```python
from build123d import *

# Parameters (mm, degrees)
BASE_W                  = 80
BASE_H                  = 101.6
BOSS_EXTRUDE1_DEPTH     = 76.2
SKETCH2_OUTSIDE_W       = 133.62
SKETCH2_OUTSIDE_H       = 108.22
CUT_EXTRUDE1_DEPTH      = 122.602138139
CUT_EXTRUDE2_DEPTH      = 122.602138139
CUT_EXTRUDE5_DEPTH      = 122.602138139
CUT_EXTRUDE5_DEPTH_BACK = 122.602138139
FILLET9_R               = 5


with BuildPart() as part:
    # Base → Boss-Extrude1 (new body)
    with BuildSketch(Plane(origin=(0, 0, 0), x_dir=(1, 0, 0), z_dir=(0, 1, 0))):
        Rectangle(BASE_W, BASE_H)
    extrude(amount=BOSS_EXTRUDE1_DEPTH)

    # Sketch2 outside → Cut-Extrude1 (cut, through all)
    with BuildSketch(Plane.ZY.offset(40)):
        with Locations((0, 38.1)):
            Rectangle(SKETCH2_OUTSIDE_W, SKETCH2_OUTSIDE_H)
        Polygon((-50.8, 0), (3.783173521, 76.2), (27.722793107, 7.014775443), (50.8, 15), (50.8, 0), align=None, mode=Mode.SUBTRACT)
    extrude(amount=-CUT_EXTRUDE1_DEPTH, mode=Mode.SUBTRACT)

    # Sketch3 → Cut-Extrude2 (cut, through all)
    with BuildSketch(Plane.ZY.offset(40)):
        Polygon((-41.426759988, 0), (22.086778061, 0), (1.39927914, 59.786633335), align=None)
    extrude(amount=-CUT_EXTRUDE2_DEPTH, mode=Mode.SUBTRACT)

    # Sketch4 → Cut-Extrude5 (cut, two sides: drawn at the far end of the back side and taken through both)
    with BuildSketch(Plane.ZY.offset(40).offset(-CUT_EXTRUDE5_DEPTH_BACK)):
        Polygon((-50.478149223, 233.014597048), (27.722793107, 7.014775443), (28.419950021, 5), (44.690435309, 5), (44.690435309, 12.88595534), (44.690435309, 252.032995353), (-49.038158805, 721.053440145), (-144.206743336, 702.035041841), align=None)
    extrude(amount=CUT_EXTRUDE5_DEPTH + CUT_EXTRUDE5_DEPTH_BACK, mode=Mode.SUBTRACT)

    # Fillet9
    # the kernel refuses this fillet: 5 mm, written as the material it takes off along each edge
    with BuildSketch(Plane(origin=(35, 65.430074367, 2.218938363), x_dir=(0, 0.3269994156125086, 0.9450245405221379), z_dir=(1, 0, 0))) as fillet9_piece_1_section:
        Polygon((0, 0), (FILLET9_R * 1.02, 0), (FILLET9_R * 1.02, -FILLET9_R * 1.97193336822), (-FILLET9_R * 0.58939542952, -FILLET9_R * 0.832474040232), align=None)
    fillet9_piece_1 = extrude(amount=FILLET9_R * 1.02, mode=Mode.PRIVATE)
    fillet9_piece_1 = fillet9_piece_1 - Plane(origin=(35, 65.430074367, 2.218938363), x_dir=(0, -0.9896165143253448, -0.14373292794121578), z_dir=(1, 0, 0)) * Sphere(FILLET9_R, mode=Mode.PRIVATE)
    add(fillet9_piece_1, mode=Mode.SUBTRACT)
    with BuildSketch(Plane(origin=(-35, 65.430074367, 2.218938363), x_dir=(0, 0.5823298395581055, -0.8129526172909656), z_dir=(-1, 0, 0))) as fillet9_piece_2_section:
        Polygon((0, 0), (FILLET9_R * 1.02, 0), (FILLET9_R * 1.02, -FILLET9_R * 1.97193336822), (-FILLET9_R * 0.58939542952, -FILLET9_R * 0.832474040232), align=None)
    fillet9_piece_2 = extrude(amount=FILLET9_R * 1.02, mode=Mode.PRIVATE)
    fillet9_piece_2 = fillet9_piece_2 - Plane(origin=(-35, 65.430074367, 2.218938363), x_dir=(0, -0.9896165143253448, -0.14373292794121578), z_dir=(-1, 0, 0)) * Sphere(FILLET9_R, mode=Mode.PRIVATE)
    add(fillet9_piece_2, mode=Mode.SUBTRACT)
    with BuildSketch(Plane(origin=(40, 67.065071445, 6.944061066), x_dir=(-1, 0, 0), z_dir=(0, -0.9450245405221379, 0.32699941561250884))) as fillet9_piece_3_section:
        with BuildLine():
            CenterArc((FILLET9_R, FILLET9_R), FILLET9_R, 180, 90)
            Line((0, FILLET9_R), (0, 0))
            Line((0, 0), (FILLET9_R, 0))
        make_face()
    fillet9_piece_3 = extrude(amount=78.175618763, mode=Mode.PRIVATE)
    fillet9_piece_3 = split(fillet9_piece_3, bisect_by=Plane(origin=(40, 5, 6.944061066), z_dir=(0, 1, 0)), keep=Keep.TOP, mode=Mode.PRIVATE)
    add(fillet9_piece_3, mode=Mode.SUBTRACT)
    with BuildSketch(Plane(origin=(40, -12.5, 50.8), x_dir=(-1, 0, 0), z_dir=(0, 1, 0))) as fillet9_piece_4:
        with BuildLine():
            CenterArc((FILLET9_R, -FILLET9_R), FILLET9_R, 90, 90)
            Line((0, -FILLET9_R), (0, 0))
            Line((0, 0), (FILLET9_R, 0))
        make_face()
    extrude(amount=40, mode=Mode.SUBTRACT)
    with BuildSketch(Plane(origin=(-57.473442698, 15, 50.8), x_dir=(0, -0.32699941561252693, -0.9450245405221316), z_dir=(1, 0, 0))) as fillet9_piece_5:
        with BuildLine():
            CenterArc((7.010644923, -4.970135785), FILLET9_R, 96.265339119, 102.821413949)
            Line((2.28552222, -6.605132863), (0, 0))
            Line((0, 0), (6.464979934, 0))
        make_face()
    extrude(amount=114.946885396, mode=Mode.SUBTRACT)
    with BuildSketch(Plane(origin=(-40, -12.5, 50.8), x_dir=(1, 0, 0), z_dir=(0, 1, 0))) as fillet9_piece_6:
        with BuildLine():
            CenterArc((FILLET9_R, FILLET9_R), FILLET9_R, 180, 90)
            Line((0, FILLET9_R), (0, 0))
            Line((0, 0), (FILLET9_R, 0))
        make_face()
    extrude(amount=40, mode=Mode.SUBTRACT)
    with BuildSketch(Plane(origin=(-40, -6.812806757, 32.507442716), x_dir=(1, 0, 0), z_dir=(0, 0.9450245405221379, -0.32699941561250884))) as fillet9_piece_7_section:
        with BuildLine():
            CenterArc((FILLET9_R, FILLET9_R), FILLET9_R, 180, 90)
            Line((0, FILLET9_R), (0, 0))
            Line((0, 0), (FILLET9_R, 0))
        make_face()
    fillet9_piece_7 = extrude(amount=78.175618763, mode=Mode.PRIVATE)
    fillet9_piece_7 = split(fillet9_piece_7, bisect_by=Plane(origin=(-40, 5, 32.507442716), z_dir=(0, 1, 0)), keep=Keep.TOP, mode=Mode.PRIVATE)
    add(fillet9_piece_7, mode=Mode.SUBTRACT)
    with BuildSketch(Plane(origin=(-40, -10.161907716, -58.079122994), x_dir=(1, 0, 0), z_dir=(0, 0.8129526172909656, 0.5823298395581055)), Plane(origin=(40, 68.341723565, -1.845824723), x_dir=(-1, 0, 0), z_dir=(0, -0.8129526172909656, -0.5823298395581055))) as fillet9_piece_8:
        with BuildLine():
            CenterArc((FILLET9_R, -FILLET9_R), FILLET9_R, 90, 90)
            Line((0, -FILLET9_R), (0, 0))
            Line((0, 0), (FILLET9_R, 0))
        make_face()
    extrude(amount=96.566060077, mode=Mode.SUBTRACT)
    with BuildSketch(Plane(origin=(-35, 76.2, 3.783173521), x_dir=(0, -0.8129526172909656, -0.5823298395581056), z_dir=(1, 0, 0))) as fillet9_piece_9:
        with BuildLine():
            CenterArc((FILLET9_R * 1.93326800806, -FILLET9_R), FILLET9_R, 90, 125.29866839)
            Line((FILLET9_R * 1.11711698822, -FILLET9_R * 1.57783865639), (0, 0))
            Line((0, 0), (FILLET9_R * 1.93326800806, 0))
        make_face()
    extrude(amount=70, mode=Mode.SUBTRACT)


solid = part.part
```
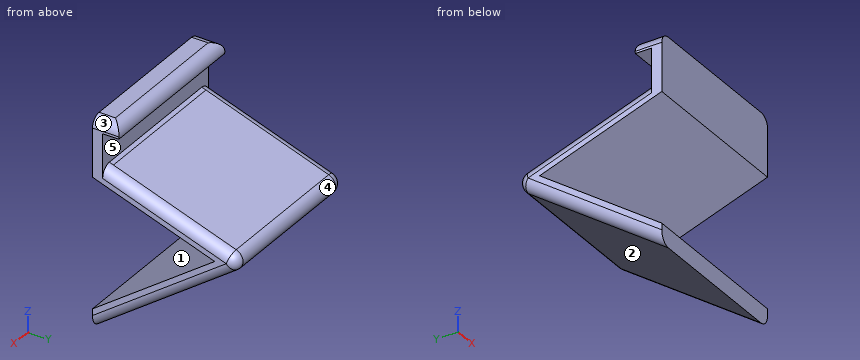
CAD build for the part. Positions are in the model's coordinates, mm. Face numbers are marked on the shaded views. A direction names the side the tool comes from. Round coordinates to 2 decimals unless told otherwise and drop trailing zeros. Loops run counter-clockwise (first coordinate to the right, second up) from the corner with the lowest first, then second, coordinate; pieces in that order, holes last. Notation, with made-up numbers: (32, 21) - (51, 21) arc R23 cw to (51, 45) - close; hole circle Ø4 at (-11, -15). An arc over 180 degrees is marked (long way). Return JSON: item names as keys, results as strings. Group by question number.
Q1. Drill centre lines: line 1 along Z through (x, y) = (-7, 11); line 2 along Z through (x, y) = (-26.5, 15.5); line 3 along Y through (x, z) = (-16, 37.5). Where is each one in solid material? Low to high. Write a range as [from, to].
Q2. Band-saw the part on B-B on z = 35. Give the cut face in (x, y).
Q3. Flat gauge pins, fed straight in: pin 1 Ø12 at (x, z) = (13.5, -17) entering from -Y; pin 2 Ø8 at (y, z) = (53, 14) entering from -X; pin 3 Ø1.5 at (x, z) = (-3, -17) entering from -Y; pin 4 Ø4 at (y, z) = (48, 17.5) entering from -X. Where does each tip first touch, or does it go through?
Q4. Band-saw the part on A-A on x = 3. Give the cut face in (y, z), plus the area to 3 significant figures.
Q5. Two-plate mould, pull along Z, no slides. Class the marked faces 3, 4 and 5: +Z half, -Z half, draft (parallel to the pull), parting line (faces both ways), or undercut.
Q6. Tool access for the marked faces 1 and 2: list every direction of +Z, -Z, +X, -X, +Y, -Y with a clear straight run to the whole face (end or side of a thin tool).
Solutions:
{
 "1": {"line 1": "z = [-42.92, -33.55], [18.28, 26.34], [44.69, 49.81]", "line 2": "z = [-39.7, -30.32], [16.72, 24.79]", "line 3": "y = [0, 5]"},
 "2": {"outline": "(-40, 0) - (40, 0) - (40, 5) - (-40, 5) - close"},
 "3": {"pin 1": "stops at y = 25.72", "pin 2": "stops at x = -38.95", "pin 3": "stops at y = 33.05", "pin 4": "passes through"},
 "4": {"outline": "(0, -50.8) - (68.34, -1.85) arc R5 ccw to (67.07, 6.94) - (5, 28.42) - (5, 44.69) - (12.89, 44.69) arc R5 ccw to (8.01, 50.8) - (0, 50.8) - (0, 22.09) - (59.79, 1.4) - (0, -41.43) - close", "area": "1,320 mm^2"},
 "5": {"face 3": "+Z half", "face 4": "parting line", "face 5": "undercut"},
 "6": {"face 1": "+X, -X, -Y", "face 2": "-Z, +X, -X, +Y"}
}
